```python
from build123d import *

# Parameters (mm, degrees)
SKETCH1_R           = 9.65
BOSS_EXTRUDE1_DEPTH = 2.5
CUT_EXTRUDE2_DEPTH  = 6
FILLET1_R           = 7.62
SKETCH3_R           = 3.175
CUT_EXTRUDE3_DEPTH  = 31.75
CUT_EXTRUDE4_DEPTH  = 6


with BuildPart() as part:
    # Sketch1 → Boss-Extrude1 (new body, symmetric)
    with BuildSketch(Plane.XY):
        with BuildLine():
            ThreePointArc((-148.66489382, -20.32), (-159.663416448, -13.97), (-159.663416448, -1.27))
            Line((-159.663416448, -1.27), (-83.131265013, 131.287574699))
            ThreePointArc((-83.131265013, 131.287574699), (-78.482742385, 135.936097327), (-72.132742385, 137.637574699))
            Line((-72.132742385, 137.637574699), (72.132742385, 137.637574699))
            ThreePointArc((72.132742385, 137.637574699), (78.482742385, 135.936097327), (83.131265013, 131.287574699))
            Line((83.131265013, 131.287574699), (159.663416448, -1.27))
            ThreePointArc((159.663416448, -1.27), (159.663416448, -13.97), (148.66489382, -20.32))
            Line((148.66489382, -20.32), (-148.66489382, -20.32))
        make_face()
        Circle(SKETCH1_R, mode=Mode.SUBTRACT)
        with Locations((-135.466666667, 0)):
            Circle(SKETCH1_R, mode=Mode.SUBTRACT)
        with Locations((135.466666667, 0)):
            Circle(SKETCH1_R, mode=Mode.SUBTRACT)
        with Locations((-67.733333333, 117.317574699)):
            Circle(SKETCH1_R, mode=Mode.SUBTRACT)
        with Locations((67.733333333, 117.317574699)):
            Circle(SKETCH1_R, mode=Mode.SUBTRACT)
    extrude(amount=BOSS_EXTRUDE1_DEPTH, both=True)

    # Sketch2 → Cut-Extrude2 (cut, through all)
    with BuildSketch(Plane.XY.offset(2.5)):
        Polygon((-17.476488174, 17.78), (-60.462836348, 94.350444874), (-104.670803308, 17.78), align=None)
        Polygon((59.840980548, 95.427530715), (1.38432688, 17.78), (104.670803308, 17.78), align=None)
    extrude(amount=-CUT_EXTRUDE2_DEPTH, mode=Mode.SUBTRACT)

    # Fillet1
    fillet1_edges = [part.edges().sort_by_distance(p)[0] for p in [
        (-17.476488174, 17.78, 0),
        (-104.670803308, 17.78, 0),
        (-60.462836348, 94.350444874, 0),
        (59.840980548, 95.427530715, 0),
        (104.670803308, 17.78, 0),
        (1.38432688, 17.78, 0),
    ]]
    fillet(fillet1_edges, radius=FILLET1_R)

    # Sketch3 → Cut-Extrude3 (cut)
    with BuildSketch(Plane.XY.offset(2.5)):
        with Locations((0, 63.5)):
            Circle(SKETCH3_R)
    extrude(amount=-CUT_EXTRUDE3_DEPTH, mode=Mode.SUBTRACT)

    # Sketch4 → Cut-Extrude4 (cut, through all)
    with BuildSketch(Plane.XY.offset(2.5)):
        with BuildLine():
            Line((-114.175443212, 29.25748078), (-82.425443212, 84.25009392))
            ThreePointArc((-82.425443212, 84.25009392), (-83.82, 89.454650708), (-89.024556788, 88.06009392))
            Line((-89.024556788, 88.06009392), (-120.774556788, 33.06748078))
            ThreePointArc((-120.774556788, 33.06748078), (-119.38, 27.862923991), (-114.175443212, 29.25748078))
        make_face()
        Polygon((-47.20148926, 112.237574699), (-27.620295809, 77.358112791), (-26.188384166, 84.842364861), (-45.769577617, 119.721826769), align=None)
        Polygon((45.769577617, 119.721826769), (26.188384166, 84.842364861), (27.620295809, 77.358112791), (47.20148926, 112.237574699), align=None)
        with BuildLine():
            Line((3.978915409, 89.950381514), (25.210877866, 116.699310593))
            ThreePointArc((25.210877866, 116.699310593), (25.806368519, 122.066920569), (21.231962456, 124.937574699))
            Line((21.231962456, 124.937574699), (-21.231962456, 124.937574699))
            ThreePointArc((-21.231962456, 124.937574699), (-25.806368519, 122.066920569), (-25.210877866, 116.699310593))
            Line((-25.210877866, 116.699310593), (-3.978915409, 89.950381514))
            ThreePointArc((-3.978915409, 89.950381514), (0, 88.028645621), (3.978915409, 89.950381514))
        make_face()
        with BuildLine():
            Line((82.425443212, 84.25009392), (114.175443212, 29.25748078))
            ThreePointArc((114.175443212, 29.25748078), (119.38, 27.862923991), (120.774556788, 33.06748078))
            Line((120.774556788, 33.06748078), (89.024556788, 88.06009392))
            ThreePointArc((89.024556788, 88.06009392), (83.82, 89.454650708), (82.425443212, 84.25009392))
        make_face()
        with BuildLine():
            Line((88.9, 3.81), (38.1, 3.81))
            ThreePointArc((38.1, 3.81), (34.29, 0), (38.1, -3.81))
            Line((38.1, -3.81), (88.9, -3.81))
            ThreePointArc((88.9, -3.81), (92.71, 0), (88.9, 3.81))
        make_face()
        with BuildLine():
            Line((-3.05, 63.5), (-3.05, 51.5))
            ThreePointArc((-3.05, 51.5), (0, 48.45), (3.05, 51.5))
            Line((3.05, 51.5), (3.05, 63.5))
            ThreePointArc((3.05, 63.5), (0, 66.55), (-3.05, 63.5))
        make_face()
        with BuildLine():
            Line((6, 78.5), (6, 38.5))
            ThreePointArc((6, 38.5), (9, 35.5), (12, 38.5))
            Line((12, 38.5), (12, 78.5))
            ThreePointArc((12, 78.5), (9, 81.5), (6, 78.5))
        make_face()
        with BuildLine():
            Line((-12, 78.5), (-12, 38.5))
            ThreePointArc((-12, 38.5), (-9, 35.5), (-6, 38.5))
            Line((-6, 38.5), (-6, 78.5))
            ThreePointArc((-6, 78.5), (-9, 81.5), (-12, 78.5))
        make_face()
    extrude(amount=-CUT_EXTRUDE4_DEPTH, mode=Mode.SUBTRACT)


solid = part.part
```
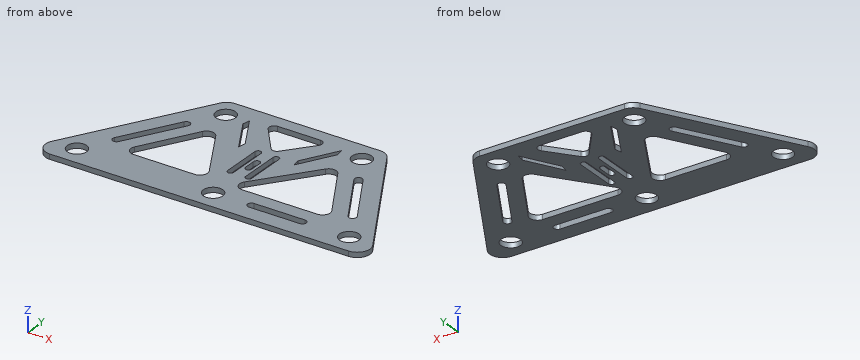
Model file for the job. Use its own axes, mm. Coordinates: 2 decimals unless noted, no trailing zeros. Order: outer loops, then holes, each group sorted by start corner. A loop starts at its lowest first (then second) coordinate and runs counter-clockwise, first axis right, second up. Notation, with made-up numbers: (37.25, 5) - (47.25, 5) arc R32 ccw to (47.25, 31) - close; hole circle Ø1 at (38.5, 18). An arc over 180 degrees is marked (long way). Return JSON: item names as keys, results as strings. Group by question number.
1) Saw through at D-D, the plane z = -0.3. Count the separate pieces of the cut face and the enclosed holes in it, plus the area to 3 significant figures.
2) Saw through at B-B, the plane x = -64. Write the cut outline in (y, z), plus the area to 3 significant figures.
3) Saw through at A-A, the plane x = 0. Write the cut outline in (y, z) (3 decimals).
4) Probe line 1 (Y direction, x = 55, z = 0.95); line 2 (X direction, y = 93.5, z = 0.8); line 3 (X direction, y = 33.5, z = -0.3). List the from-to ranges inside material, lowest first. Write a range as from..to.
5) Flat gauge pins, fed straight in: P1, Ø1, axis at y = 10, z = -1, coming from the +X side; P2, Ø4, axis at x = 0, y = 63.5, coming from the +Z side; P3, Ø2.5, axis at y = 58, z = 0.5, coming from the -X side; P4, Ø1.5, axis at y = 68, z = -0.5, coming from the -X side. Where does each tip first touch, or does it go through?
6) Saw through at C-C, the plane y = 100. Write the cut outline in (x, z), plus the area to 3 significant figures.
Values found:
{
 "1": {"separate pieces": "1", "enclosed holes": "16", "area": "27,000 mm²"},
 "2": {"outline": "(-20.32, -2.5) - (17.78, -2.5) - (17.78, 2.5) - (-20.32, 2.5) - close; (85.75, -2.5) - (108.42, -2.5) - (108.42, 2.5) - (85.75, 2.5) - close; (126.22, -2.5) - (137.64, -2.5) - (137.64, 2.5) - (126.22, 2.5) - close", "area": "361 mm²"},
 "3": {"outline": "(-20.32, -2.5) - (-9.65, -2.5) - (-9.65, 2.5) - (-20.32, 2.5) - close; (9.65, -2.5) - (48.45, -2.5) - (48.45, 2.5) - (9.65, 2.5) - close; (66.675, -2.5) - (88.029, -2.5) - (88.029, 2.5) - (66.675, 2.5) - close; (124.938, -2.5) - (137.638, -2.5) - (137.638, 2.5) - (124.938, 2.5) - close"},
 "4": {"line 1": "y = -20.32..-3.81, 3.81..17.78, 88.13..137.64", "line 2": "x = -104.95..-36.68, -31.05..-6.8, 6.8..31.05, 36.68..104.95", "line 3": "x = -139.59..-120.52, -111.73..-95.59, -26.3..13.22, 95.59..111.73, 120.52..139.59"},
 "5": {"P1": "stops at x = 153.45", "P2": "passes through", "P3": "stops at x = -126.17", "P4": "stops at x = -120.1"},
 "6": {"outline": "(-101.2, -2.5) - (-40.33, -2.5) - (-40.33, 2.5) - (-101.2, 2.5) - close; (-34.7, -2.5) - (-11.96, -2.5) - (-11.96, 2.5) - (-34.7, 2.5) - close; (11.96, -2.5) - (34.7, -2.5) - (34.7, 2.5) - (11.96, 2.5) - close; (40.33, -2.5) - (101.2, -2.5) - (101.2, 2.5) - (40.33, 2.5) - close", "area": "836 mm²"}
}
